Design review of the part shown in the three views and the two pictorial views. Dimensions are in mm from the part's minimum x, y and z. A direction names the side the tool comes from. Give positions to 0.01 mm unless a question says otherwise; leave off trailing zeros. Write each loop counter-clockwise with the first axis right and the second up, starting at its lowest first coordinate (ties: lowest second). Pieces come first, ordered by that corner, then holes. Notation, with made-up numbers: (22, 12.25) -> (60, 12.25) arc R30 cw to (60, 42.25) -> close; hole circle Ø9 at (5.25, 15.5). An arc over 180 degrees is marked (long way). Use CSV: the item, a comma, the result in double quotes.
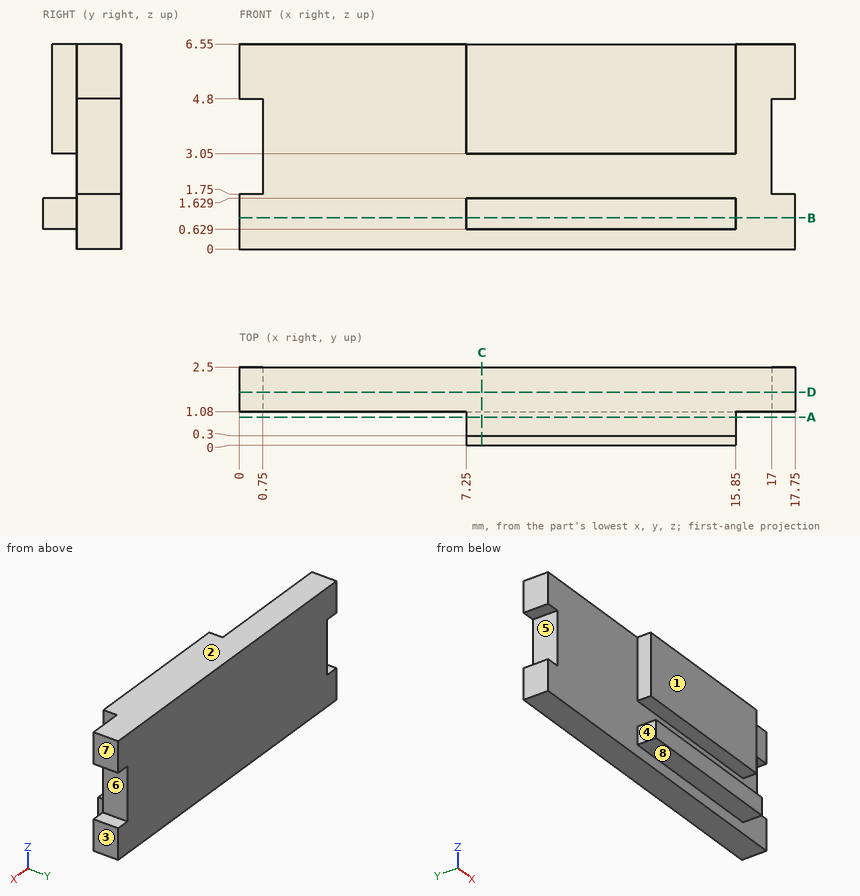
Q1. Machinability: for the marked faces 1, 2, 3, 4 and 5, which of the approach directions +Z, -Z, +X, -X, +Y, -Y give a long, thin tool a straight path to every point of the face, cutting with its end or side? Answer none if there is none.
Derived:
face 1,"+Z, +X, -X, -Y"
face 2,"+Z, +X, -X, +Y, -Y"
face 3,"+Z, -Z, +X, +Y, -Y"
face 4,"+Z, -Z, -X, -Y"
face 5,"-X, +Y, -Y"
Q2. Consider section A-A (y = 0.9). Write out the cut boundary in (x, z).
Derived:
outline,"(7.25, 0.63) -> (15.85, 0.63) -> (15.85, 1.63) -> (7.25, 1.63) -> close; (7.25, 3.05) -> (15.85, 3.05) -> (15.85, 6.55) -> (7.25, 6.55) -> close"
Q3. Consider section D-D (y = 1.7). Write out the cut boundary in (x, z).
Derived:
outline,"(0, 0) -> (17.75, 0) -> (17.75, 1.75) -> (17, 1.75) -> (17, 4.8) -> (17.75, 4.8) -> (17.75, 6.55) -> (0, 6.55) -> (0, 4.8) -> (0.75, 4.8) -> (0.75, 1.75) -> (0, 1.75) -> close"
Q4. Consider section C-C (x = 7.75). Write out the cut boundary in (y, z).
Derived:
outline,"(0, 0.63) -> (1.08, 0.63) -> (1.08, 0) -> (2.5, 0) -> (2.5, 6.55) -> (0.3, 6.55) -> (0.3, 3.05) -> (1.08, 3.05) -> (1.08, 1.63) -> (0, 1.63) -> close"
Q5. The part is to be moulded in two halves that separate along Z. For the marked faces 6, 7 and 8, say which applies: pulls with the +Z half, pulls with the -Z half, needs draft (parallel to the pull), parting line crosses it, or undercut.
Derived:
face 6,"undercut"
face 7,"needs draft"
face 8,"pulls with the -Z half"
Q6. Consider section B-B (z = 1). Write out the cut boundary in (x, y).
Derived:
outline,"(0, 1.08) -> (7.25, 1.08) -> (7.25, 0) -> (15.85, 0) -> (15.85, 1.08) -> (17.75, 1.08) -> (17.75, 2.5) -> (0, 2.5) -> close"
Q7. To check wall thickness, follow probe 1 along Z at (x, y) = (15.25, 0.85); probe 2 along X at (y, z) = (2.05, 3.25); probe 3 along Y at (x, z) = (12.5, 2.5). State the ranges of each line that lie inside material, in increasing order.
Derived:
probe 1,"z = 0.63 to 1.63, 3.05 to 6.55"
probe 2,"x = 0.75 to 17"
probe 3,"y = 1.08 to 2.5"
Q8. Insertion check: pin 1 (0.9 mm diameter, centred on y = 0.5, z = 5.5, fed in from +X); pin 2 (0.8 mm diameter, centred on y = 0.5, z = 1.5, fed in from -X); pin 3 (2 mm diameter, centred on x = 6.5, z = 4.5, fed in from -Y). Each pin has a flat end and moves straight along its axis. Give the tip position at first contact, or say it passes through.
Derived:
pin 1,"stops at x = 15.85"
pin 2,"stops at x = 7.25"
pin 3,"stops at y = 0.3"
